The figure shows three views and two pictorial views of one solid part (mm, origin at its lowest corner). Answer the questions. A direction names the side the tool comes from. Give positions to 0.01 mm unless a question says otherwise; leave off trailing zeros. Loops run counter-clockwise (first coordinate to the right, second up) from the corner with the lowest first, then second, coordinate; pieces in that order, holes last. Notation, with made-up numbers: M 11,60.5 L 67,60.5 A8 ccw 67,66.5 Z; hole C -14,66.5 d3. An arc over 180 degrees is marked long. Answer in a Markdown table with one row per item. Add a question column.
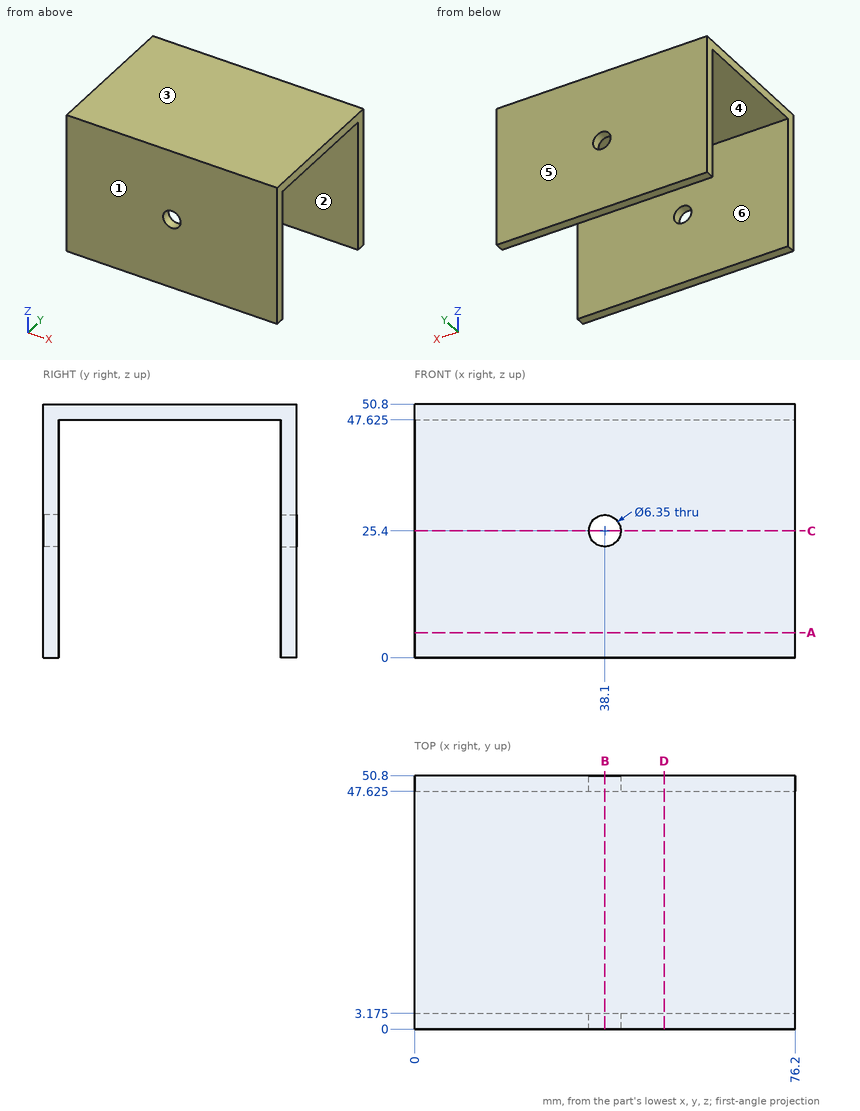
(1) Consider line 1 along Z through (x, y) = (38.1, 0.85) (3 decimals); line 2 along Y through (x, z) = (37.5, 30.5) (3 decimals); line 3 along X through (y, z) = (49.8, 25.4) (3 decimals). Determine where each line is inside the solid, lowest interval first. Write a range as from..to.
(2) This flat-tipped pin is pushed along its axis until it touches: P1, Ø2, axis at x = 32, y = 11, coming from the -Z side (3 decimals). Where does it stop, or does it pass through?
(3) Section B-B, the plane x = 38.1 is taken. Determine the outline of the cut face in (y, z) (3 decimals), and give its area (3 significant figures).
(4) Section C-C, the plane z = 25.4 is taken. Determine the outline of the cut face in (x, y) (3 decimals).
(5) Section A-A, the plane z = 5 is taken. Determine the outline of the cut face in (x, y) (3 decimals).
(6) Which of the six approach directions +Z, -Z, +X, -X, +Y, -Y give full straight-line access (tool end or side, diameter ignored) to the marked faces 1 and 2?
(7) The mould has two halves that part along Y. Classify the marked faces 3, 4, 5 and 6: pulls with the +Y half, pulls with the -Y half, needs draft (parallel to the pull), parting line crosses it, or undercut.
(8) Section D-D, the plane x = 50 is taken. Determine the outline of the cut face in (y, z) (3 decimals), and give its area (3 significant figures).
Numbers:
| question | item | result |
|---|---|---|
| 1 | line 1 | z = 0..22.225, 28.575..50.8 |
| 1 | line 2 | y = 0..3.175, 47.625..50.8 |
| 1 | line 3 | x = 0..34.925, 41.275..76.2 |
| 2 | P1 | stops at z = 47.625 |
| 3 | outline | M 0,0 L 3.175,0 L 3.175,22.225 L 0,22.225 Z; M 0,28.575 L 3.175,28.575 L 3.175,47.625 L 47.625,47.625 L 47.625,28.575 L 50.8,28.575 L 50.8,50.8 L 0,50.8 Z; M 47.625,0 L 50.8,0 L 50.8,22.225 L 47.625,22.225 Z |
| 3 | area | 423 mm² |
| 4 | outline | M 0,0 L 34.925,0 L 34.925,3.175 L 0,3.175 Z; M 0,47.625 L 34.925,47.625 L 34.925,50.8 L 0,50.8 Z; M 41.275,0 L 76.2,0 L 76.2,3.175 L 41.275,3.175 Z; M 41.275,47.625 L 76.2,47.625 L 76.2,50.8 L 41.275,50.8 Z |
| 5 | outline | M 0,0 L 76.2,0 L 76.2,3.175 L 0,3.175 Z; M 0,47.625 L 76.2,47.625 L 76.2,50.8 L 0,50.8 Z |
| 6 | face 1 | +Z, -Z, +X, -X, -Y |
| 6 | face 2 | -Z, +X, -X |
| 7 | face 3 | needs draft |
| 7 | face 4 | undercut |
| 7 | face 5 | pulls with the +Y half |
| 7 | face 6 | undercut |
| 8 | outline | M 0,0 L 3.175,0 L 3.175,47.625 L 47.625,47.625 L 47.625,0 L 50.8,0 L 50.8,50.8 L 0,50.8 Z |
| 8 | area | 464 mm² |
